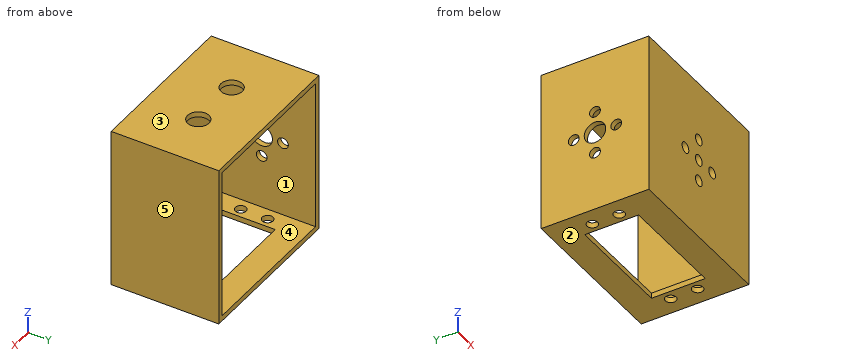
from build123d import *

# Parameters (mm, degrees)
IZIM2_W                     = 60
IZIM2_H                     = 40
Y_KSEKLIK_EKSTR_ZYON1_DEPTH = 60
BO_ALTMA1_T                 = -2
KES_EKSTR_ZYON2_REACH       = 95.808
IZIM4_R                     = 2
IZIM4_W                     = 40
IZIM4_H                     = 20
KES_EKSTR_ZYON3_REACH       = 95.808
IZIM5_R                     = 2
KES_EKSTR_ZYON4_REACH       = 95.808
IZIM6_R                     = 4
KES_EKSTR_ZYON5_REACH       = 95.808
IZIM7_R                     = 4
IZIM7_R_2                   = 2


with BuildPart() as part:
    # Çizim2 → Yükseklik-Ekstrüzyon1 (new body)
    with BuildSketch(Plane.XY):
        with Locations((30, 20)):
            Rectangle(IZIM2_W, IZIM2_H)
    extrude(amount=Y_KSEKLIK_EKSTR_ZYON1_DEPTH)

    # İç Boşaltma1
    bo_altma1_openings = [part.faces().sort_by_distance(p)[0] for p in [
        (30, 40, 30),
    ]]
    offset(amount=BO_ALTMA1_T, openings=bo_altma1_openings, kind=Kind.INTERSECTION)

    # Çizim4 → Kes-Ekstrüzyon2 (cut, up to next)
    with BuildSketch(Plane(origin=(0, 0, 0), x_dir=(-1, 0, 0), z_dir=(0, 0, -1)), mode=Mode.PRIVATE) as kes_ekstr_zyon2_sk1:
        with Locations((-53.5, 25)):
            Circle(IZIM4_R)
    kes_ekstr_zyon2_tool1 = extrude(kes_ekstr_zyon2_sk1.sketch, amount=-KES_EKSTR_ZYON2_REACH, mode=Mode.PRIVATE) & part.part
    # Çizim4 → Kes-Ekstrüzyon2 (cut, up to next)
    with BuildSketch(Plane(origin=(0, 0, 0), x_dir=(-1, 0, 0), z_dir=(0, 0, -1)), mode=Mode.PRIVATE) as kes_ekstr_zyon2_sk2:
        with Locations((-53.5, 15)):
            Circle(IZIM4_R)
    kes_ekstr_zyon2_tool2 = extrude(kes_ekstr_zyon2_sk2.sketch, amount=-KES_EKSTR_ZYON2_REACH, mode=Mode.PRIVATE) & part.part
    # Çizim4 → Kes-Ekstrüzyon2 (cut, up to next)
    with BuildSketch(Plane(origin=(0, 0, 0), x_dir=(-1, 0, 0), z_dir=(0, 0, -1)), mode=Mode.PRIVATE) as kes_ekstr_zyon2_sk3:
        with Locations((-6.5, 15)):
            Circle(IZIM4_R)
    kes_ekstr_zyon2_tool3 = extrude(kes_ekstr_zyon2_sk3.sketch, amount=-KES_EKSTR_ZYON2_REACH, mode=Mode.PRIVATE) & part.part
    # Çizim4 → Kes-Ekstrüzyon2 (cut, up to next)
    with BuildSketch(Plane(origin=(0, 0, 0), x_dir=(-1, 0, 0), z_dir=(0, 0, -1)), mode=Mode.PRIVATE) as kes_ekstr_zyon2_sk4:
        with Locations((-6.5, 25)):
            Circle(IZIM4_R)
    kes_ekstr_zyon2_tool4 = extrude(kes_ekstr_zyon2_sk4.sketch, amount=-KES_EKSTR_ZYON2_REACH, mode=Mode.PRIVATE) & part.part
    # Çizim4 → Kes-Ekstrüzyon2 (cut, up to next)
    with BuildSketch(Plane(origin=(0, 0, 0), x_dir=(-1, 0, 0), z_dir=(0, 0, -1)), mode=Mode.PRIVATE) as kes_ekstr_zyon2_sk5:
        with Locations((-30, 20)):
            Rectangle(IZIM4_W, IZIM4_H)
    kes_ekstr_zyon2_tool5 = extrude(kes_ekstr_zyon2_sk5.sketch, amount=-KES_EKSTR_ZYON2_REACH, mode=Mode.PRIVATE) & part.part
    add(kes_ekstr_zyon2_tool1.solids().sort_by_distance((53.5, 25, 0))[0], mode=Mode.SUBTRACT)
    add(kes_ekstr_zyon2_tool2.solids().sort_by_distance((53.5, 15, 0))[0], mode=Mode.SUBTRACT)
    add(kes_ekstr_zyon2_tool3.solids().sort_by_distance((6.5, 15, 0))[0], mode=Mode.SUBTRACT)
    add(kes_ekstr_zyon2_tool4.solids().sort_by_distance((6.5, 25, 0))[0], mode=Mode.SUBTRACT)
    add(kes_ekstr_zyon2_tool5.solids().sort_by_distance((30, 20, 0))[0], mode=Mode.SUBTRACT)

    # Çizim5 → Kes-Ekstrüzyon3 (cut, up to next)
    with BuildSketch(Plane.XZ, mode=Mode.PRIVATE) as kes_ekstr_zyon3_sk1:
        with Locations(Location((30, 30, 0), (0, 0, 270))):
            Circle(IZIM5_R)
    kes_ekstr_zyon3_tool1 = extrude(kes_ekstr_zyon3_sk1.sketch, amount=-KES_EKSTR_ZYON3_REACH, mode=Mode.PRIVATE) & part.part
    # Çizim5 → Kes-Ekstrüzyon3 (cut, up to next)
    with BuildSketch(Plane.XZ, mode=Mode.PRIVATE) as kes_ekstr_zyon3_sk2:
        with Locations(Location((38, 30, 0), (0, 0, 270))):
            Circle(IZIM5_R)
    kes_ekstr_zyon3_tool2 = extrude(kes_ekstr_zyon3_sk2.sketch, amount=-KES_EKSTR_ZYON3_REACH, mode=Mode.PRIVATE) & part.part
    # Çizim5 → Kes-Ekstrüzyon3 (cut, up to next)
    with BuildSketch(Plane.XZ, mode=Mode.PRIVATE) as kes_ekstr_zyon3_sk3:
        with Locations(Location((30, 38, 0), (0, 0, 270))):
            Circle(IZIM5_R)
    kes_ekstr_zyon3_tool3 = extrude(kes_ekstr_zyon3_sk3.sketch, amount=-KES_EKSTR_ZYON3_REACH, mode=Mode.PRIVATE) & part.part
    # Çizim5 → Kes-Ekstrüzyon3 (cut, up to next)
    with BuildSketch(Plane.XZ, mode=Mode.PRIVATE) as kes_ekstr_zyon3_sk4:
        with Locations(Location((30, 22, 0), (0, 0, 90))):
            Circle(IZIM5_R)
    kes_ekstr_zyon3_tool4 = extrude(kes_ekstr_zyon3_sk4.sketch, amount=-KES_EKSTR_ZYON3_REACH, mode=Mode.PRIVATE) & part.part
    # Çizim5 → Kes-Ekstrüzyon3 (cut, up to next)
    with BuildSketch(Plane.XZ, mode=Mode.PRIVATE) as kes_ekstr_zyon3_sk5:
        with Locations(Location((22, 30, 0), (0, 0, 90))):
            Circle(IZIM5_R)
    kes_ekstr_zyon3_tool5 = extrude(kes_ekstr_zyon3_sk5.sketch, amount=-KES_EKSTR_ZYON3_REACH, mode=Mode.PRIVATE) & part.part
    add(kes_ekstr_zyon3_tool1.solids().sort_by_distance((30, 0, 30))[0], mode=Mode.SUBTRACT)
    add(kes_ekstr_zyon3_tool2.solids().sort_by_distance((38, 0, 30))[0], mode=Mode.SUBTRACT)
    add(kes_ekstr_zyon3_tool3.solids().sort_by_distance((30, 0, 38))[0], mode=Mode.SUBTRACT)
    add(kes_ekstr_zyon3_tool4.solids().sort_by_distance((30, 0, 22))[0], mode=Mode.SUBTRACT)
    add(kes_ekstr_zyon3_tool5.solids().sort_by_distance((22, 0, 30))[0], mode=Mode.SUBTRACT)

    # Çizim6 → Kes-Ekstrüzyon4 (cut, up to next)
    with BuildSketch(Plane.XY.offset(60), mode=Mode.PRIVATE) as kes_ekstr_zyon4_sk1:
        with Locations((20, 20)):
            Circle(IZIM6_R)
    kes_ekstr_zyon4_tool1 = extrude(kes_ekstr_zyon4_sk1.sketch, amount=-KES_EKSTR_ZYON4_REACH, mode=Mode.PRIVATE) & part.part
    # Çizim6 → Kes-Ekstrüzyon4 (cut, up to next)
    with BuildSketch(Plane.XY.offset(60), mode=Mode.PRIVATE) as kes_ekstr_zyon4_sk2:
        with Locations(Location((40, 20, 0), (0, 0, 180))):
            Circle(IZIM6_R)
    kes_ekstr_zyon4_tool2 = extrude(kes_ekstr_zyon4_sk2.sketch, amount=-KES_EKSTR_ZYON4_REACH, mode=Mode.PRIVATE) & part.part
    add(kes_ekstr_zyon4_tool1.solids().sort_by_distance((20, 20, 60))[0], mode=Mode.SUBTRACT)
    add(kes_ekstr_zyon4_tool2.solids().sort_by_distance((40, 20, 60))[0], mode=Mode.SUBTRACT)

    # Çizim7 → Kes-Ekstrüzyon5 (cut, up to next)
    with BuildSketch(Plane.ZY, mode=Mode.PRIVATE) as kes_ekstr_zyon5_sk1:
        with Locations((30, 20)):
            Circle(IZIM7_R)
    kes_ekstr_zyon5_tool1 = extrude(kes_ekstr_zyon5_sk1.sketch, amount=-KES_EKSTR_ZYON5_REACH, mode=Mode.PRIVATE) & part.part
    # Çizim7 → Kes-Ekstrüzyon5 (cut, up to next)
    with BuildSketch(Plane.ZY, mode=Mode.PRIVATE) as kes_ekstr_zyon5_sk2:
        with Locations((22, 20)):
            Circle(IZIM7_R_2)
    kes_ekstr_zyon5_tool2 = extrude(kes_ekstr_zyon5_sk2.sketch, amount=-KES_EKSTR_ZYON5_REACH, mode=Mode.PRIVATE) & part.part
    # Çizim7 → Kes-Ekstrüzyon5 (cut, up to next)
    with BuildSketch(Plane.ZY, mode=Mode.PRIVATE) as kes_ekstr_zyon5_sk3:
        with Locations(Location((38, 20, 0), (0, 0, 180))):
            Circle(IZIM7_R_2)
    kes_ekstr_zyon5_tool3 = extrude(kes_ekstr_zyon5_sk3.sketch, amount=-KES_EKSTR_ZYON5_REACH, mode=Mode.PRIVATE) & part.part
    # Çizim7 → Kes-Ekstrüzyon5 (cut, up to next)
    with BuildSketch(Plane.ZY, mode=Mode.PRIVATE) as kes_ekstr_zyon5_sk4:
        with Locations((30, 27.898318077)):
            Circle(IZIM7_R_2)
    kes_ekstr_zyon5_tool4 = extrude(kes_ekstr_zyon5_sk4.sketch, amount=-KES_EKSTR_ZYON5_REACH, mode=Mode.PRIVATE) & part.part
    # Çizim7 → Kes-Ekstrüzyon5 (cut, up to next)
    with BuildSketch(Plane.ZY, mode=Mode.PRIVATE) as kes_ekstr_zyon5_sk5:
        with Locations(Location((30, 12.101681923, 0), (0, 0, 180))):
            Circle(IZIM7_R_2)
    kes_ekstr_zyon5_tool5 = extrude(kes_ekstr_zyon5_sk5.sketch, amount=-KES_EKSTR_ZYON5_REACH, mode=Mode.PRIVATE) & part.part
    add(kes_ekstr_zyon5_tool1.solids().sort_by_distance((0, 20, 30))[0], mode=Mode.SUBTRACT)
    add(kes_ekstr_zyon5_tool2.solids().sort_by_distance((0, 20, 22))[0], mode=Mode.SUBTRACT)
    add(kes_ekstr_zyon5_tool3.solids().sort_by_distance((0, 20, 38))[0], mode=Mode.SUBTRACT)
    add(kes_ekstr_zyon5_tool4.solids().sort_by_distance((0, 27.898318, 30))[0], mode=Mode.SUBTRACT)
    add(kes_ekstr_zyon5_tool5.solids().sort_by_distance((0, 12.101682, 30))[0], mode=Mode.SUBTRACT)


solid = part.part
Here's how the part is built. I have some questions about the finished solid (model axes, mm). Face numbers are marked on the shaded views. A direction names the side the tool comes from. Coordinates: 2 decimals unless noted, no trailing zeros. Write each loop counter-clockwise with the first axis right and the second up, starting at its lowest first coordinate (ties: lowest second). Pieces come first, ordered by that corner, then holes.
1) If I drill on line 1 (Y direction, x = 1, z = 30); line 2 (X direction, y = 1, z = 30); line 3 (Z direction, x = 30.5, y = 31.5), over which ranges is the centre line in solid material (lowest first)?
Filled in:
line 1: y = 0 to 10.1, 14.1 to 16, 24 to 25.9, 29.9 to 40
line 2: x = 0 to 20, 24 to 28, 32 to 36, 40 to 60
line 3: z = 0 to 2, 58 to 60
2) If we section it at D-D (y = 9): List the corners of the cut face in (x, z) for me.
Filled in:
outline: (0, 0) - (60, 0) - (60, 60) - (0, 60) - close; hole (2, 2) - (58, 2) - (58, 58) - (2, 58) - close
3) Which directions (+Z, -Z, +X, -X, +Y, -Y) give clear straight access to the entire face, cutting with the end or side of a thin tool? Please do the marked faces 4 and 5.
Filled in:
face 4: +Y
face 5: +Z, -Z, +X, +Y, -Y
4) If we section it at A-A (y = 20): Count the separate pieces of the cut face and the enclosed holes in it, plus the area to 3 significant figures.
Filled in:
separate pieces: 6
enclosed holes: 0
area: 320 mm2
5) I'm going to push flat-ended pins straight in: pin 1 (12 mm diameter, centred on x = 19.5, y = 31.5, fed in from -Z); pin 2 (3.5 mm diameter, centred on x = 6.5, y = 15, fed in from -Z); pin 3 (1.5 mm diameter, centred on x = 39, z = 28, fed in from +Y); pin 4 (3 mm diameter, centred on x = 22, z = 30, fed in from -Y). Where does each tip first touch, or does it pass through?
Filled in:
pin 1: stops at z = 0
pin 2: stops at z = 58
pin 3: stops at y = 2
pin 4: passes through
6) Thinking about a two-plate mould opening in Z: for the marked faces 1, 2 and 3, which applies, +Z half, -Z half, draft (parallel to the pull), parting line (faces both ways), or undercut?
Filled in:
face 1: undercut
face 2: -Z half
face 3: +Z half
7) If we section it at C-C (x = 30): List the corners of the cut face in (y, z) for me.
Filled in:
outline: (0, 0) - (10, 0) - (10, 2) - (2, 2) - (2, 20) - (0, 20) - close; (0, 24) - (2, 24) - (2, 28) - (0, 28) - close; (0, 32) - (2, 32) - (2, 36) - (0, 36) - close; (0, 40) - (2, 40) - (2, 58) - (40, 58) - (40, 60) - (0, 60) - close; (30, 0) - (40, 0) - (40, 2) - (30, 2) - close
